```python
from build123d import *

# Parameters (mm, degrees)
F0_R          = 48.895
F0_R_2        = 47.625
F1_DEPTH      = 3.175
F2_R          = 1.5875
F3_DEPTH      = 48.896
F3_DEPTH_BACK = 88.97111
F4_R          = 1.5875
F5_DEPTH      = 48.8960001


with BuildPart() as f1:
    # F0 (on Front) → F1 (new body, symmetric)
    with BuildSketch(Plane.XZ):
        Circle(F0_R)
        Circle(F0_R_2, mode=Mode.SUBTRACT)
    extrude(amount=F1_DEPTH, both=True)

    # F2 (on Right) → F3 (cut, two sides)
    with BuildSketch(Plane.YZ) as f3_sk:
        Circle(F2_R)
    extrude(amount=-F3_DEPTH, mode=Mode.SUBTRACT)
    extrude(f3_sk.sketch, amount=F3_DEPTH_BACK, mode=Mode.SUBTRACT)

    # F4 (on Top) → F5 (cut, through all)
    with BuildSketch(Plane.XY):
        Circle(F4_R)
    extrude(amount=-F5_DEPTH, mode=Mode.SUBTRACT)


solid = f1.part
```
Verification items for the finished model (mm, model axes). A direction names the side the tool comes from. Round coordinates to 2 decimals unless told otherwise and drop trailing zeros. Order: outer loops, then holes, each group sorted by start corner. A loop starts at its lowest first (then second) coordinate and runs counter-clockwise, first axis right, second up. Notation, with made-up numbers: (-8.5, 79) -> (27.5, 79) arc R7 cw to (27.5, 91) -> close; hole circle Ø2 at (23.5, 4.5). An arc over 180 degrees is marked (long way). Put each result on its own line as item: value. Start each with the question number.
(1) Material ranges on line 1 along Y through (x, z) = (0, -48.35) (1 decimal); line 2 along X through (y, z) = (-2.5, -0.5); line 3 along X through (y, z) = (1, -39.5), recorded low to high.
(2) Section check A-A (z = 0). Enter the section's corners in (x, y) (1 decimal).
(3) Section check D-D (y = 0). State how many separate pieces and enclosed holes the cut face has, then the cut area to 3 significant figures.
(4) Section check B-B (x = 0). Enter the section's corners in (y, z) (1 decimal).
(5) Section check C-C (x = 19.5). Enter the section's corners in (y, z) (3 decimals).
(6) Draft check along Z on faces 1 (the face through (-48.24, 0.85, 1.34)), 2 (the face through (-10.599, -0.044, -47.732)), 3 (the face through (11, 3.175, -47)). Enter one of: +Z half, -Z half, draft (parallel to the pull), parting line (faces both ways), or undercut.
(7) Depth check by flat-ended pin: pin 1 Ø2 at (x, y) = (11.5, -2) entering from +Z; pin 2 Ø1.5 at (y, z) = (-0.5, 9.5) entering from -X. Enter the tip coordinate at first touch or a pass-through.
(8) Tool access check on faces 4 (the face through (-0.34, -1.55, -48.24)), 5 (the face through (48.24, 0.85, 1.34)). Record the directions out of +Z, -Z, +X, -X, +Y, -Y that give a thin tool (end or side, any length) a straight path to the whole face; none if there is none.
Completed:
1. line 1: y = -3.2 to -1.6, 1.6 to 3.2
1. line 2: x = -48.89 to -47.62, 47.62 to 48.89
1. line 3: x = -28.82 to -26.61, 26.61 to 28.82
2. outline: (-48.9, -3.2) -> (-47.6, -3.2) -> (-47.6, -1.6) -> (-48.9, -1.6) -> close; (-48.9, 1.6) -> (-47.6, 1.6) -> (-47.6, 3.2) -> (-48.9, 3.2) -> close; (47.6, -3.2) -> (48.9, -3.2) -> (48.9, -1.6) -> (47.6, -1.6) -> close; (47.6, 1.6) -> (48.9, 1.6) -> (48.9, 3.2) -> (47.6, 3.2) -> close
3. separate pieces: 3
3. enclosed holes: 0
3. area: 373 mm2
4. outline: (-3.2, -48.9) -> (-1.6, -48.9) -> (-1.6, -47.6) -> (-3.2, -47.6) -> close; (-3.2, 47.6) -> (3.2, 47.6) -> (3.2, 48.9) -> (-3.2, 48.9) -> close; (1.6, -48.9) -> (3.2, -48.9) -> (3.2, -47.6) -> (1.6, -47.6) -> close
5. outline: (-3.175, -44.838) -> (3.175, -44.838) -> (3.175, -43.45) -> (-3.175, -43.45) -> close; (-3.175, 43.45) -> (3.175, 43.45) -> (3.175, 44.838) -> (-3.175, 44.838) -> close
6. face 1: undercut
6. face 2: parting line
6. face 3: draft
7. pin 1: stops at z = 47.75
7. pin 2: stops at x = -48.11
8. face 4: -Z
8. face 5: +X, -X
